Verification items for the finished model (mm, model axes). A direction names the side the tool comes from. Round coordinates to 2 decimals unless told otherwise and drop trailing zeros. Write each loop counter-clockwise with the first axis right and the second up, starting at its lowest first coordinate (ties: lowest second). Pieces come first, ordered by that corner, then holes. Notation, with made-up numbers: (-17.75, 21) - (18.25, 21) arc R18 cw to (18.25, 43) - close; hole circle Ø4 at (48, 84). An arc over 180 degrees is marked (long way). Answer as a JSON object with one key per item and string values.
```python
from build123d import *

# Parameters (mm, degrees)
SKETCH_1_R               = 17.5
EXTRUDE_1_DEPTH          = 200
EXTRUDE_1_TAPER          = 2
EXTRUDE_2_DEPTH          = 12.5
EXTRUDE_2_DRAFT          = -25
CUT_EXTRUDE_1_DEPTH      = 12.5
SKETCH_5_R               = 1.55
CUT_EXTRUDE_2_DEPTH      = 203.439460302
CHAMFER_1_SIZE           = 3
CHAMFER_1_SIZE2          = 3.812436427
PATTERN_CIRCULAR_2_COUNT = 3
EXTRUDE_3_DEPTH          = 13
SKETCH_12_R              = 1.25
CUT_EXTRUDE_3_DEPTH      = 82.605855603
CUT_EXTRUDE_4_DEPTH      = 82.605855603
CUT_EXTRUDE_4_DEPTH_BACK = 82.605855603
SKETCH_13_R              = 1.25
CHAMFER_3_SIZE           = 12
CHAMFER_3_SIZE2          = 6.769076267
CHAMFER_4_SIZE           = 0.8
CHAMFER_4_SIZE2          = 1.385640646


with BuildPart() as part:
    # 草图1 → 凸台-拉伸1 (new body)
    with BuildSketch(Plane(origin=(0, 0, 0), x_dir=(1, 0, 0), z_dir=(0, 1, 0))):
        Circle(SKETCH_1_R)
    extrude(amount=EXTRUDE_1_DEPTH, taper=EXTRUDE_1_TAPER)


with BuildPart() as extrude_2_tool:
    # 凸台-拉伸2: read off the stored shape, not the designer's step
    # 凸台-拉伸2 outline → 凸台-拉伸2 (with draft: the straight prism first)
    with BuildSketch(Plane.XZ.offset(12.5)):
        with BuildLine():
            Line((-2.078845727, -1.817738728), (14.578845727, -1.817738728))
            Line((14.578845727, -1.817738728), (14.578845727, 18.212421591))
            ThreePointArc((14.578845727, 18.212421591), (6.735850314, 22.335249349), (-2.078845727, 23.236037601))
            Line((-2.078845727, 23.236037601), (-2.078845727, -1.817738728))
        make_face()
    extrude(amount=-EXTRUDE_2_DEPTH)
    # 凸台-拉伸2: the draft: its side faces are tilted about the plane it starts from
    extrude_2_sides = [extrude_2_tool.faces().sort_by_distance(p)[0] for p in [
        (-2.078845727, -6.25, 10.709149437),
        (6.25, -6.25, -1.817738728),
        (14.578845727, -6.25, 8.197341431),
        (6.735850314, -6.25, 22.335249349),
    ]]
    draft(extrude_2_sides, Plane.XZ.offset(12.5), EXTRUDE_2_DRAFT)


with BuildPart() as part_1:
    add(part.part)

    # 凸台-拉伸2: add extrude_2_tool
    add(extrude_2_tool.part)

    # 草图4 → 切除-拉伸1 (cut)
    with BuildSketch(Plane.XZ.offset(12.5)):
        Polygon((8.75, 15.155444566), (8.75, 21.625737975), (8.75, 22.625737975), (15.578845727, 22.625737975), (15.578845727, -2.817738728), (8.75, -2.817738728), (8.75, 4.011106999), align=None)
        Polygon((3.75, 17.093492914), (3.75, 23.025475955), (3.75, 24.025475955), (-3.078845727, 24.025475955), (-3.078845727, -2.817738728), (3.75, -2.817738728), (3.75, 4.011106999), align=None)
    extrude(amount=-CUT_EXTRUDE_1_DEPTH, mode=Mode.SUBTRACT)

    # 草图5 → 切除-拉伸2 (cut, through all)
    with BuildSketch(Plane.ZY.offset(-3.75)):
        with Locations((15, -8)):
            Circle(SKETCH_5_R)
        with BuildLine():
            Line((4.011106999, 0), (12.214361758, -10.95327183))
            ThreePointArc((12.214361758, -10.95327183), (16.970472378, -12.122462651), (19.047673538, -7.68705616))
            Line((19.047673538, -7.68705616), (17.093492914, 0))
            Line((17.093492914, 0), (24.025475955, 0))
            Line((24.025475955, 0), (24.025475955, -13.5))
            Line((24.025475955, -13.5), (-2.817738728, -13.5))
            Line((-2.817738728, -13.5), (-2.817738728, 0))
            Line((-2.817738728, 0), (4.011106999, 0))
        make_face()
    extrude(amount=-CUT_EXTRUDE_2_DEPTH, mode=Mode.SUBTRACT)

    # 倒角1
    chamfer_1_edges = [part_1.edges().sort_by_distance(p)[0] for p in [
        (6.25, 0, 4.011106999),
    ]]
    chamfer_1_side = [part_1.faces().sort_by_distance(p)[0] for p in [
        (-0.420899726, 0, -0.691089635),
    ]]
    chamfer(chamfer_1_edges, length=CHAMFER_1_SIZE, length2=CHAMFER_1_SIZE2, reference=chamfer_1_side[0])


with BuildPart() as pattern_circular_2_1:
    # 阵列(圆周)2: pattern copy
    add(part_1.part.rotate(Axis((0, 0, 0), (0, 1, 0)), 1 * 360 / PATTERN_CIRCULAR_2_COUNT))


with BuildPart() as pattern_circular_2_2:
    # 阵列(圆周)2: pattern copy
    add(part_1.part.rotate(Axis((0, 0, 0), (0, 1, 0)), 2 * 360 / PATTERN_CIRCULAR_2_COUNT))


with BuildPart() as pattern_circular_2_1_1:
    add(pattern_circular_2_1.part)

    # Combine 1: read off the stored shape, not the designer's step
    # Combine 1: union 阵列(圆周)2_2, part
    add(pattern_circular_2_2.part)
    add(part_1.part)

    # 草图10 → 切除-旋转1 (revolve, cut)
    with BuildSketch(Plane(origin=(0, 0, 0), x_dir=(0, 0, -1), z_dir=(1, 0, 0))):
        Polygon((0, 2), (15.629061281, 2), (13.027463954, 63.5), (13.027463954, 76.5), (23.027463954, 76.5), (23.027463954, 210), (0, 210), align=None)
    revolve(axis=Axis((0, 0, 0), (0, 1, 0)), mode=Mode.SUBTRACT)

    # 草图11 → 凸台-拉伸3 (add)
    with BuildSketch(Plane(origin=(0, 76.5, 0), x_dir=(1, 0, 0), z_dir=(0, 1, 0))):
        Polygon((13.928012544, 0), (13.928012544, -1.5), (11.027463954, -1.5), (11.027463954, 1.5), (13.928012544, 1.5), align=None)
    extrude(amount=-EXTRUDE_3_DEPTH)

    # 草图12 → 切除-拉伸3 (cut, through all)
    with BuildSketch(Plane(origin=(0, 0, 0), x_dir=(0, 0, -1), z_dir=(1, 0, 0))):
        with Locations((0, 71.31)):
            Circle(SKETCH_12_R)
    extrude(amount=-CUT_EXTRUDE_3_DEPTH, mode=Mode.SUBTRACT)

    # 草图13 → 切除-拉伸4 (cut, two sides: drawn at the far end of the back side and taken through both)
    with BuildSketch(Plane.XY.offset(-CUT_EXTRUDE_4_DEPTH_BACK)):
        with Locations((0, 71.31)):
            Circle(SKETCH_13_R)
    extrude(amount=CUT_EXTRUDE_4_DEPTH + CUT_EXTRUDE_4_DEPTH_BACK, mode=Mode.SUBTRACT)

    # 倒角3
    chamfer_3_edges = [pattern_circular_2_1_1.edges().sort_by_distance(p)[0] for p in [
        (0, 2, 15.629061281),
    ]]
    chamfer_3_side = [pattern_circular_2_1_1.faces().sort_by_distance(p)[0] for p in [
        (0, 2, 0),
    ]]
    chamfer(chamfer_3_edges, length=CHAMFER_3_SIZE, length2=CHAMFER_3_SIZE2, reference=chamfer_3_side[0])

    # 倒角4
    chamfer_4_edges = [pattern_circular_2_1_1.edges().sort_by_distance(p)[0] for p in [
        (-13.027463954, 76.5, 0),
    ]]
    chamfer_4_side = [pattern_circular_2_1_1.faces().sort_by_distance(p)[0] for p in [
        (7.204573044, 76.5, 12.47868656),
    ]]
    chamfer(chamfer_4_edges, length=CHAMFER_4_SIZE, length2=CHAMFER_4_SIZE2, reference=chamfer_4_side[0])


solid = pattern_circular_2_1_1.part
```
1. Cross-section at C-C (y = 32). Record the boundary of the cut face in (x, z), plus the area to 3 significant figures.
Completed:
{"outline": "circle Ø32.77 at (0, 0); hole circle Ø28.72 at (0, 0)", "area": "195 mm^2"}
2. Go/stop test with flat-tipped pins: pin 1 (10 mm diameter, centred on y = -7.5, z = 9, fed in from +X); pin 2 (8 mm diameter, centred on x = 0, z = 0.5, fed in from +Y); pin 3 (1.5 mm diameter, centred on y = 73, z = 0.5, fed in from -X); pin 4 (1.9 mm diameter, centred on y = -8, z = 15, fed in from -X). Record where each tip stops, or that it passes through.
Completed:
{"pin 1": "stops at x = 8.75", "pin 2": "stops at y = 2.5", "pin 3": "stops at x = -14.97", "pin 4": "passes through"}
3. Cross-section at D-D (y = 45). Record the boundary of the cut face in (x, z), plus the area to 3 significant figures.
Completed:
{"outline": "circle Ø31.86 at (0, 0); hole circle Ø27.62 at (0, 0)", "area": "198 mm^2"}
4. Access from +Z, -Z, +X, -X, +Y, -Y to the whole of each face (thin tool, end or side, straight path). Record for faces 1 (the face through (6.219, -4.949, -13.694)), 2 (the face through (8.75, -5, 12)), 3 (the face through (6.215, -1.547, 3.691)), 4 (the face through (11.027, 70, 0)).
Completed:
{"face 1": "-Z, -X, -Y", "face 2": "+Z, +X, -Y", "face 3": "+X, -Y", "face 4": "+Y"}
5. Material ranges on probe 1 along Y at (x, z) = (4.5, -4.5); probe 2 along X at (y, z) = (11.5, 6); probe 3 along X at (y, z) = (31, 7), recorded low to high. Write a range as from..to.
Completed:
{"probe 1": "y = 0..3.58", "probe 2": "x = -16.01..-14, 14..16.01", "probe 3": "x = -14.85..-12.59, 12.59..14.85"}
6. Mould release check, pull along Y, two halves, no side actions. Record for faces 5 (the face through (3.75, -5, 12)), 6 (the face through (-15.807, -9.513, -1.95)), 7 (the face through (-18.68, -4.75, -4.25)), 8 (the face through (0.672, 72.364, 13.996)): released by +Y, released by -Y, zero draft, split by the parting line, or undercut.
Completed:
{"face 5": "zero draft", "face 6": "undercut", "face 7": "released by +Y", "face 8": "undercut"}
7. Cross-section at A-A (x = 0). Record the boundary of the cut face in (y, z).
Completed:
{"outline": "(-2.33, -10.1) - (0, -10.1) - (0, -17.5) - (70.06, -15.05) - (70.06, -13.03) - (63.5, -13.03) - (8.76, -15.34) - (2, -3.63) - (2, 3.63) - (8.76, 15.34) - (63.5, 13.03) - (70.06, 13.03) - (70.06, 15.05) - (0, 17.5) - (0, -4.33) - (-0.67, -4.33) - close; (72.56, -14.97) - (76.5, -14.83) - (76.5, -13.83) - (75.11, -13.03) - (72.56, -13.03) - close; (72.56, 13.03) - (75.11, 13.03) - (76.5, 13.83) - (76.5, 14.83) - (72.56, 14.97) - close"}
